Could you check a few things on this model? Use its own coordinates, in mm. Give positions to 0.01 mm unless a question says otherwise; leave off trailing zeros. Write each loop counter-clockwise with the first axis right and the second up, starting at its lowest first coordinate (ties: lowest second). Pieces come first, ordered by that corner, then holes. Notation, with made-up numbers: M -24.5,44 L 12.5,44 A26 ccw 12.5,61 Z; hole C 47.25,89 d2. An arc over 180 degrees is marked long. One line per item, written item: value.
```python
from build123d import *

# Parameters (mm, degrees)
SKETCH_1_W      = 695
SKETCH_1_H      = 70
EXTRUDE_1_DEPTH = 4
EXTRUDE_2_DEPTH = 3
EXTRUDE_3_DEPTH = 3


with BuildPart() as part:
    # Эскиз1 → Бобышка-Вытянуть1 (new body)
    with BuildSketch(Plane.XY):
        with Locations((347.5, -5.198933607)):
            Rectangle(SKETCH_1_W, SKETCH_1_H)
    extrude(amount=EXTRUDE_1_DEPTH)

    # Эскиз2 → Бобышка-Вытянуть2 (add)
    with BuildSketch(Plane.XZ.offset(40.198933607)):
        with BuildLine():
            Line((47, 4), (147, 4))
            ThreePointArc((147, 4), (149, 2), (147, 0))
            Line((147, 0), (47, 0))
            ThreePointArc((47, 0), (45, 2), (47, 4))
        make_face()
        with BuildLine():
            Line((217, 4), (317, 4))
            ThreePointArc((317, 4), (319, 2), (317, 0))
            Line((317, 0), (217, 0))
            ThreePointArc((217, 0), (215, 2), (217, 4))
        make_face()
        with BuildLine():
            Line((387, 4), (487, 4))
            ThreePointArc((487, 4), (489, 2), (487, 0))
            Line((487, 0), (387, 0))
            ThreePointArc((387, 0), (385, 2), (387, 4))
        make_face()
        with BuildLine():
            Line((557, 4), (657, 4))
            ThreePointArc((657, 4), (659, 2), (657, 0))
            Line((657, 0), (557, 0))
            ThreePointArc((557, 0), (555, 2), (557, 4))
        make_face()
    extrude(amount=EXTRUDE_2_DEPTH)

    # Эскиз3 → Бобышка-Вытянуть3 (add)
    with BuildSketch(Plane.ZY):
        with BuildLine():
            Line((4, 20), (4, -20))
            ThreePointArc((4, -20), (2, -22), (0, -20))
            Line((0, -20), (0, 20))
            ThreePointArc((0, 20), (2, 22), (4, 20))
        make_face()
    extrude(amount=EXTRUDE_3_DEPTH)


solid = part.part
```
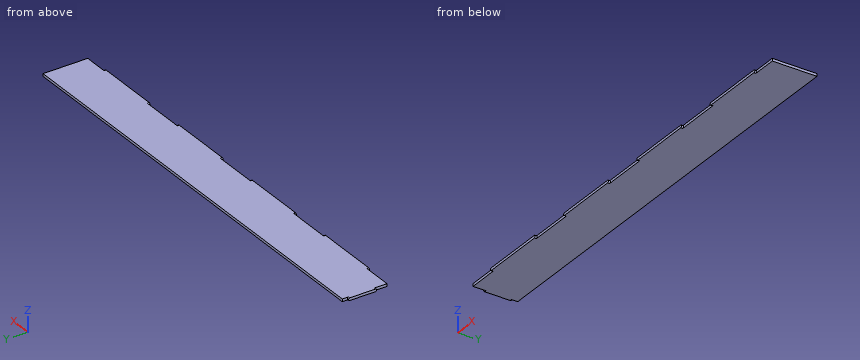
1) I'm going to push flat-ended pins straight in: pin 1 (1.2 mm diameter, centred on x = 198.5, z = 2.5, fed in from -Y); pin 2 (1.2 mm diameter, centred on y = 26, z = 1.5, fed in from -X). Where does each tip first touch, or does it pass through?
Outcome:
pin 1: stops at y = -40.2
pin 2: stops at x = 0
2) If we section it at B-B, the plane x = 209: Write out the boundary of the cut face in (y, z), then the cut area to 3 significant figures.
Outcome:
outline: M -40.2,0 L 29.8,0 L 29.8,4 L -40.2,4 Z
area: 280 mm^2
3) If we section it at A-A, the plane z = 2: Write out the boundary of the cut face in (x, y), then the cut area to 3 significant figures.
Outcome:
outline: M -3,-22 L 0,-22 L 0,-40.2 L 45,-40.2 L 45,-43.2 L 149,-43.2 L 149,-40.2 L 215,-40.2 L 215,-43.2 L 319,-43.2 L 319,-40.2 L 385,-40.2 L 385,-43.2 L 489,-43.2 L 489,-40.2 L 555,-40.2 L 555,-43.2 L 659,-43.2 L 659,-40.2 L 695,-40.2 L 695,29.8 L 0,29.8 L 0,22 L -3,22 Z
area: 50,000 mm^2
4) Please list where these lines run through material, in increasing order: L1, parallel to X at y = -34.5, z = 3.1; L2, parallel to Y at x = 383.5, z = 1.8. Write a range as from..to.
Outcome:
L1: x = 0..695
L2: y = -40.2..29.8
